from build123d import *

# Parameters (mm, degrees)
PAD_DEPTH    = 5
SKETCH001_W  = 4
SKETCH001_H  = 10
PAD001_DEPTH = 12
POCKET_DEPTH = 2


with BuildPart() as part:
    # Sketch → Pad (new body)
    with BuildSketch(Plane.XY):
        Polygon((-35, 10), (35, 10), (45, 0), (35, -10), (-35, -10), (-45, 0), align=None)
    extrude(amount=PAD_DEPTH)

    # Sketch001 (on Face8 of Pad) → Pad001 (join)
    with BuildSketch(Plane.XY.offset(5)):
        with Locations((-13, 0)):
            Rectangle(SKETCH001_W, SKETCH001_H)
    extrude(amount=PAD001_DEPTH)

    # Sketch002 (on Face12 of Pad001) → Pocket (cut)
    with BuildSketch(Plane(origin=(0, 5, 0), x_dir=(-1, 0, 0), z_dir=(0, 1, 0))):
        with BuildLine():
            Line((-3.4, 17), (3.4, 17))
            Line((3.4, 17), (2.6, 7.2))
            ThreePointArc((-2.6, 7.2), (0, 4.803596), (2.6, 7.2))
            Line((-3.4, 17), (-2.6, 7.2))
        make_face()
    extrude(amount=-POCKET_DEPTH, mode=Mode.SUBTRACT)


solid = part.part
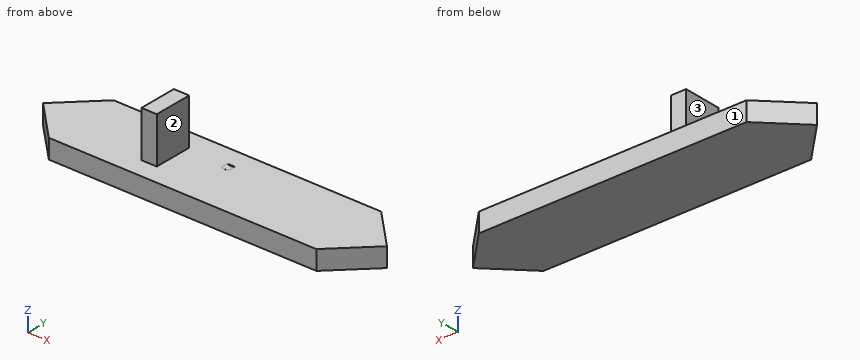
The model under review builds one solid part; all positions refer to its coordinate system, in mm. Face numbers are marked on the shaded views. A direction names the side the tool comes from. Round coordinates to 2 decimals unless told otherwise and drop trailing zeros. Loops run counter-clockwise (first coordinate to the right, second up) from the corner with the lowest first, then second, coordinate; pieces in that order, holes last. Notation, with made-up numbers: (-20.5, -20) -> (-15.5, -20) arc R15 ccw to (-15.5, -9) -> close; hole circle Ø9 at (64.5, -28). An arc over 180 degrees is marked (long way). Write item = value, one per line. Start each with the question number.
Item 1: Take a section at D-D on y = 4. Give the boundary of the cut face in (x, z).
Item 2: To check wall thickness, follow L1, parallel to Z at x = 10, y = 4.25; L2, parallel to X at y = -3.5, z = 13.75; L3, parallel to Y at x = 40, z = 2.5. State the ranges of each line that lie inside material, in increasing order.
Item 3: Take a section at C-C on z = 3. Give the boundary of the cut face in (x, y), plus the area to 3 significant figures.
Item 4: Take a section at A-A on y = -2. Give the boundary of the cut face in (x, z).
Item 5: For the marked faces 1, 2 and 3, list the 3-axis set-ups (+Z, -Z, +X, -X, +Y, -Y) from which the entire face can be reached by the end or side of a thin tool; tool diameter is ignored.
Item 6: Take a section at B-B on x = -36. Give the boundary of the cut face in (y, z), plus the area to 3 significant figures.
Item 7: Insertion check: pin 1 (6 mm diameter, centred on x = -17, z = 12.5, fed in from -Y); pin 2 (8 mm diameter, centred on y = -1, z = 15, fed in from -X); pin 3 (1 mm diameter, centred on x = 34, y = -6.5, fed in from +Z). Each pin has a flat end and moves straight along its axis. Give the tip position at first contact, or say it passes through.
Result:
q1.outline = (-41, 0) -> (41, 0) -> (41, 5) -> (0.99, 5) arc R2.61 cw to (-0.99, 5) -> (-11, 5) -> (-11, 17) -> (-15, 17) -> (-15, 5) -> (-41, 5) -> close
q2.L1 = 0 to 5
q2.L2 = -15 to -11
q2.L3 = -5 to 5
q3.outline = (-45, 0) -> (-35, -10) -> (35, -10) -> (45, 0) -> (35, 10) -> (-35, 10) -> close
q3.area = 1,600 mm²
q4.outline = (-43, 0) -> (43, 0) -> (43, 5) -> (-11, 5) -> (-11, 17) -> (-15, 17) -> (-15, 5) -> (-43, 5) -> close
q5.face_1 = +Z, -Z, +X, -X, +Y
q5.face_2 = +Z, +X, +Y, -Y
q5.face_3 = +Z, -X, +Y, -Y
q6.outline = (-9, 0) -> (9, 0) -> (9, 5) -> (-9, 5) -> close
q6.area = 90.0 mm²
q7.pin_1 = -5
q7.pin_2 = -15
q7.pin_3 = 5
